Model file for the job. Use its own axes, mm. Round coordinates to 2 decimals unless told otherwise and drop trailing zeros. Write each loop counter-clockwise with the first axis right and the second up, starting at its lowest first coordinate (ties: lowest second). Pieces come first, ordered by that corner, then holes. Notation, with made-up numbers: (61.25, -26.5) - (110.25, -26.5) arc R13 ccw to (110.25, -19.5) - close; hole circle Ø2 at (-6, 70.25). An arc over 180 degrees is marked (long way). One line per item, written item: value.
from build123d import *

# Parameters (mm, degrees)
SKETCH1_R           = 2
SKETCH1_R_2         = 1.5875
BOSS_EXTRUDE1_DEPTH = 1
SKETCH2_W           = 41.754758497
SKETCH2_H           = 54.729261875
SKETCH2_W_2         = 10.192494114
SKETCH2_H_2         = 69.784905138
SKETCH2_W_3         = 27.032266999
SKETCH2_H_3         = 25.038083368
SKETCH2_W_4         = 11.965101787
SKETCH2_H_4         = 38.554216868
SKETCH2_W_5         = 19.055532475
SKETCH2_H_5         = 12.851405623
CUT_EXTRUDE1_DEPTH  = 2


with BuildPart() as part:
    # Sketch1 → Boss-Extrude1 (new body)
    with BuildSketch(Plane.XY):
        with BuildLine():
            Line((61.109996011, 41.935724429), (61.109996011, -18.064275571))
            ThreePointArc((61.109996011, -18.064275571), (16.109996011, -63.064275571), (-28.890003989, -18.064275571))
            Line((-28.890003989, -18.064275571), (-28.890003989, 41.935724429))
            Line((-28.890003989, 41.935724429), (61.109996011, 41.935724429))
        make_face()
        with Locations((37.609996011, -41.564275571)):
            Circle(SKETCH1_R, mode=Mode.SUBTRACT)
        with Locations((-5.390003989, -41.564275571)):
            Circle(SKETCH1_R, mode=Mode.SUBTRACT)
        with Locations((1.984996011, -25.564275571)):
            Circle(SKETCH1_R, mode=Mode.SUBTRACT)
        with Locations((-9.950003989, 2.691836123)):
            Circle(SKETCH1_R_2, mode=Mode.SUBTRACT)
        with Locations((40.849996011, -12.548163877)):
            Circle(SKETCH1_R_2, mode=Mode.SUBTRACT)
        with Locations((42.119996011, 35.711836123)):
            Circle(SKETCH1_R_2, mode=Mode.SUBTRACT)
        with Locations((-9.950003989, 30.631836123)):
            Circle(SKETCH1_R_2, mode=Mode.SUBTRACT)
    extrude(amount=BOSS_EXTRUDE1_DEPTH)

    # Sketch2 → Cut-Extrude1 (cut, through all)
    with BuildSketch(Plane.XY.offset(1)):
        with Locations((16.947060745, 9.488348719)):
            Rectangle(SKETCH2_W, SKETCH2_H)
        with Locations((-18.677429553, 3.843922739)):
            Rectangle(SKETCH2_W_2, SKETCH2_H_2)
        with Locations((16.947060745, -42.471213668)):
            Rectangle(SKETCH2_W_3, SKETCH2_H_3)
        with Locations((49.346389863, 12.147260227)):
            Rectangle(SKETCH2_W_4, SKETCH2_H_4)
        with Locations((45.801174519, -27.293260477)):
            Rectangle(SKETCH2_W_5, SKETCH2_H_5)
    extrude(amount=-CUT_EXTRUDE1_DEPTH, mode=Mode.SUBTRACT)


solid = part.part
1. Band-saw the part on C-C on x = 34. Write the cut outline in (y, z), plus the area to 3 significant figures.
Report:
outline: (-59.36, 0) - (-17.88, 0) - (-17.88, 1) - (-59.36, 1) - close; (36.85, 0) - (41.94, 0) - (41.94, 1) - (36.85, 1) - close
area: 46.6 mm²
2. Band-saw the part on B-B on x = 46. Write the cut outline in (y, z).
Report:
outline: (-51.7, 0) - (-33.72, 0) - (-33.72, 1) - (-51.7, 1) - close; (-20.87, 0) - (-7.13, 0) - (-7.13, 1) - (-20.87, 1) - close; (31.42, 0) - (41.94, 0) - (41.94, 1) - (31.42, 1) - close
3. Drop a flat-ended pin along its axis: pin 1 (0.5 mm diameter, centred on x = 51, z = 0.5, fed in from -Y). Give the stop position or say it passes through.
Report:
pin 1: y = -46.79
4. Band-saw the part on D-D on z = 0.75. State how many separate pieces and enclosed holes the cut face has, plus the area to 3 significant figures.
Report:
separate pieces: 1
enclosed holes: 12
area: 4,130 mm²
5. Wall check: probe 1 along X at (y, z) = (26, 0.5); probe 2 along Y at (x, z) = (49, 0.7); probe 3 along Y at (x, z) = (11, 0.3). Give the ranges that are in metal, low to high. Write a range as [from, to].
Report:
probe 1: [-28.89, -23.77], [-13.58, -3.93], [37.82, 43.36], [55.33, 61.11]
probe 2: [-48.78, -33.72], [-20.87, -7.13], [31.42, 41.94]
probe 3: [-62.77, -54.99], [-29.95, -17.88], [36.85, 41.94]
6. Mould opens along X. For faces 1 (the face through (3.06, -23.88, 0.49)), 2 (the face through (17.1, -63.053, 0.493)), 3 (the face through (17, -21, 1)) say: released by +X, released by -X, zero draft, split by the parting line, or undercut.
Report:
face 1: undercut
face 2: split by the parting line
face 3: zero draft
7. Band-saw the part on A-A on y = -9. Write the cut outline in (x, z), plus the area to 3 significant figures.
Report:
outline: (-28.89, 0) - (-23.77, 0) - (-23.77, 1) - (-28.89, 1) - close; (-13.58, 0) - (-3.93, 0) - (-3.93, 1) - (-13.58, 1) - close; (37.82, 0) - (61.11, 0) - (61.11, 1) - (37.82, 1) - close
area: 38.1 mm²
